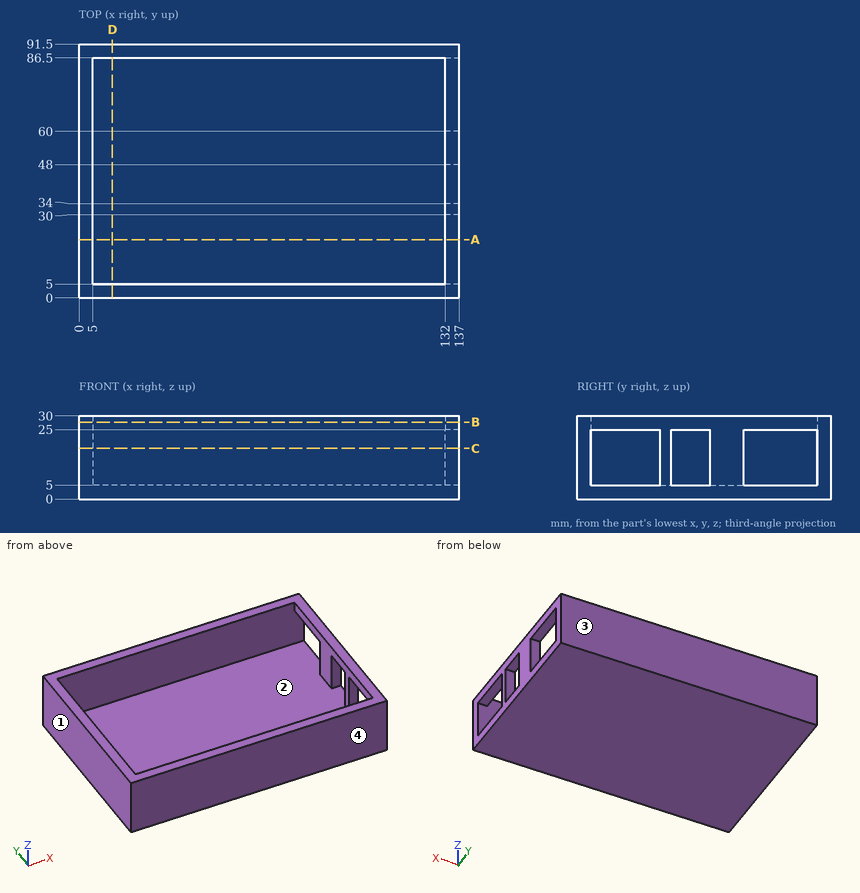
Input: dimensioned drawing with shaded views. Units: mm. Origin: part minimum x, y, z. Give positions to 0.01 mm unless a question says otherwise; leave off trailing zeros. Write each loop counter-clockwise with the first axis right and the second up, starting at its lowest first coordinate (ties: lowest second). Pieces come first, ordered by that corner, then holes. Notation, with made-up numbers: M 60.5,4 L 67.5,4 A14 cw 67.5,28 Z; hole C -23.5,-7 d4. An arc over 180 degrees is marked long. Return JSON: item names as keys, results as strings. Group by question number.
1) Cut plane D-D, the plane x = 12. Output: boundary loops of the cut face in (y, z), plus the area to 4 significant figures.
2) Cut plane A-A, the plane y = 21. Output: boundary loops of the cut face in (x, z), plus the area to 3 significant figures.
3) Material intervals for line 1 along Y through (x, z) = (51.5, 11.5); line 2 along X through (y, z) = (52, 20.75); line 3 along Z through (x, y) = (25, 68), sorted ascending. Write a range as [from, to].
4) Cut plane C-C, the plane z = 18.25. Output: boundary loops of the cut face in (x, y), plus the area to 3 significant figures.
5) Cut plane B-B, the plane z = 27.75. Output: boundary loops of the cut face in (x, y), plus the area to 4 significant figures.
6) Pin query (flat end, axial travel): P1, Ø10, axis at x = 40.5, y = 10.5, coming from the +Z side; P2, Ø12, axis at y = 68, z = 13, coming from the +X side. Return the tip coordinate at first contact, or that it passes through.
7) Pull-direction query (Y, two-part tool) for the marked faces 1, 2, 3 and 4; classes: pulls with the +Y half, pulls with the -Y half, needs draft (parallel to the pull), parting line crosses it, or undercut.
Recorded:
{
 "1": {"outline": "M 0,0 L 91.5,0 L 91.5,30 L 86.5,30 L 86.5,5 L 5,5 L 5,30 L 0,30 Z", "area": "707.5 mm²"},
 "2": {"outline": "M 0,0 L 137,0 L 137,5 L 5,5 L 5,30 L 0,30 Z; M 132,25 L 137,25 L 137,30 L 132,30 Z", "area": "835 mm²"},
 "3": {"line 1": "y = [0, 5], [86.5, 91.5]", "line 2": "x = [0, 5], [132, 137]", "line 3": "z = [0, 5]"},
 "4": {"outline": "M 0,0 L 137,0 L 137,5 L 5,5 L 5,86.5 L 137,86.5 L 137,91.5 L 0,91.5 Z; M 132,30 L 137,30 L 137,34 L 132,34 Z; M 132,48 L 137,48 L 137,60 L 132,60 Z", "area": "1,860 mm²"},
 "5": {"outline": "M 0,0 L 137,0 L 137,91.5 L 0,91.5 Z; hole M 5,5 L 132,5 L 132,86.5 L 5,86.5 Z", "area": "2,185 mm²"},
 "6": {"P1": "stops at z = 5", "P2": "stops at x = 5"},
 "7": {"face 1": "needs draft", "face 2": "undercut", "face 3": "pulls with the +Y half", "face 4": "pulls with the -Y half"}
}
